Build history of the part. All positions in model axes, mm. Face numbers are marked on the shaded views. Coordinates: 2 decimals unless noted, no trailing zeros. Order: outer loops, then holes, each group sorted by start corner. A loop starts at its lowest first (then second) coordinate and runs counter-clockwise, first axis right, second up. Notation, with made-up numbers: (87.5, 23.25) - (97.5, 23.25) arc R15 cw to (97.5, 28.25) - close; hole circle Ø2 at (39, 57.5). An arc over 180 degrees is marked (long way). Write each question's results on one line, items separated by ' | '.
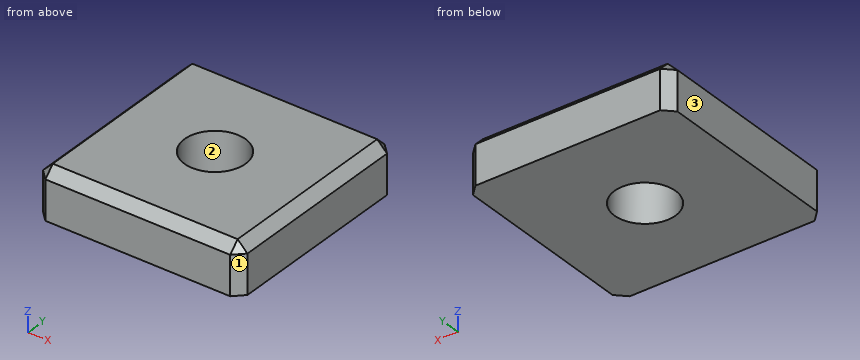
from build123d import *

# Parameters (mm, degrees)
ESQUISSE2_W                  = 20.8
ESQUISSE2_H                  = 20.8
BOSS_EXTRU_1_DEPTH           = 5
ENL_V_MAT_EXTRU_1_DEPTH      = 30.837560222
ENL_V_MAT_EXTRU_1_DEPTH_BACK = 30.837560222
ESQUISSE4_R                  = 3.1
CHANFREIN1_SIZE              = 1


with BuildPart() as part:
    # Esquisse2 → Boss.-Extru.1 (new body)
    with BuildSketch(Plane.XY):
        with Locations((10.4, 10.4)):
            Rectangle(ESQUISSE2_W, ESQUISSE2_H)
    extrude(amount=BOSS_EXTRU_1_DEPTH)

    # Esquisse4 → Enlèv. mat.-Extru.1 (cut, two sides: drawn at the far end of the back side and taken through both)
    with BuildSketch(Plane.XY.offset(5).offset(-ENL_V_MAT_EXTRU_1_DEPTH_BACK)):
        with Locations((10.4, 10.4)):
            Circle(ESQUISSE4_R)
    extrude(amount=ENL_V_MAT_EXTRU_1_DEPTH + ENL_V_MAT_EXTRU_1_DEPTH_BACK, mode=Mode.SUBTRACT)

    # Chanfrein1
    chanfrein1_edges = [part.edges().sort_by_distance(p)[0] for p in [
        (20.8, 10.4, 5),
        (10.4, 20.8, 5),
        (0, 10.4, 5),
        (0, 20.8, 2.5),
        (20.8, 20.8, 2.5),
        (20.8, 0, 2.5),
        (0, 0, 2.5),
        (10.4, 0, 5),
    ]]
    chamfer(chanfrein1_edges, length=CHANFREIN1_SIZE)


solid = part.part
1. Band-saw the part on A-A on y = 10.4. Give the cut face in (x, z), then the cut area to 3 significant figures.
Solved:
outline: (0, 0) - (7.3, 0) - (7.3, 5) - (1, 5) - (0, 4) - close; (13.5, 0) - (20.8, 0) - (20.8, 4) - (19.8, 5) - (13.5, 5) - close | area: 72.0 mm2
2. Two-plate mould, pull along Y, no slides. Class the marked faces 1, 2 and 3: +Y half, -Y half, draft (parallel to the pull), parting line (faces both ways), or undercut.
Solved:
face 1: -Y half | face 2: undercut | face 3: draft
3. Band-saw the part on B-B on z = 3.1. Give the cut face in (x, y).
Solved:
outline: (0, 1) - (1, 0) - (19.8, 0) - (20.8, 1) - (20.8, 19.8) - (19.8, 20.8) - (1, 20.8) - (0, 19.8) - close; hole circle Ø6.2 at (10.4, 10.4)
4. Probe line 1 (Y direction, x = 10.4, z = 3.2); line 2 (Y direction, x = 9.5, z = 0.8). List the from-to ranges inside material, lowest first.
Solved:
line 1: y = 0 to 7.3, 13.5 to 20.8 | line 2: y = 0 to 7.43, 13.37 to 20.8
